The model under review builds one solid part; all positions refer to its coordinate system, in mm. A direction names the side the tool comes from. Coordinates: 2 decimals unless noted, no trailing zeros. Write each loop counter-clockwise with the first axis right and the second up, starting at its lowest first coordinate (ties: lowest second). Pieces come first, ordered by that corner, then holes.
```python
from build123d import *

# Parameters (mm, degrees)
BOSS_EXTRUDE1_DEPTH = 5
CUT_EXTRUDE1_DEPTH  = 3
FILLET2_R           = 1
FILLET3_R           = 1
FILLET4_R           = 3
LPATTERN1_COUNT     = 2
LPATTERN1_PITCH     = 70
BOSS_EXTRUDE2_REACH = 80.869
SKETCH3_W           = 51.273928048
SKETCH3_H           = 5


with BuildPart() as part:
    # Sketch1 → Boss-Extrude1 (new, symmetric)
    with BuildSketch(Plane.XY):
        with BuildLine():
            Line((25.636964024, -25.75), (25.636964024, -2))
            Line((25.636964024, -2), (17.636964024, -2))
            ThreePointArc((17.636964024, -2), (0, -17.75), (-17.636964024, -2))
            Line((-17.636964024, -2), (-25.636964024, -2))
            Line((-25.636964024, -2), (-25.636964024, -25.75))
            Line((-25.636964024, -25.75), (25.636964024, -25.75))
        make_face()
    extrude(amount=BOSS_EXTRUDE1_DEPTH, both=True)

    # Sketch2 → Cut-Extrude1 (cut, symmetric)
    with BuildSketch(Plane.XY):
        Polygon((25.636964024, -2), (21.636964024, -7.712592027), (25.636964024, -18.702501705), align=None)
    cut_extrude1 = extrude(amount=CUT_EXTRUDE1_DEPTH, both=True, mode=Mode.SUBTRACT)

    # Mirror4: Cut-Extrude1 across plane
    add(cut_extrude1.mirror(Plane(origin=(0, 0, 0), x_dir=(0, 0, 1), z_dir=(1, 0, 0))), mode=Mode.SUBTRACT)

    # Fillet2
    fillet2_edges = [part.edges().sort_by_distance(p)[0] for p in [
        (25.636964024, -2, 0),
        (-25.636964024, -2, 0),
    ]]
    fillet(fillet2_edges, radius=FILLET2_R)

    # Fillet3
    fillet3_edges = [part.edges().sort_by_distance(p)[0] for p in [
        (25.636964024, -2, 4),
        (-25.636964024, -2, 4),
        (25.636964024, -2, -4),
        (-25.636964024, -2, -4),
    ]]
    fillet(fillet3_edges, radius=FILLET3_R)

    # Fillet4
    fillet4_edges = [part.edges().sort_by_distance(p)[0] for p in [
        (-17.636964024, -2, 0),
        (17.636964024, -2, 0),
    ]]
    fillet(fillet4_edges, radius=FILLET4_R)


with BuildPart() as lpattern1_1:
    # LPattern1: pattern copy
    add(part.part.moved(Location(Vector(0, 0, 1) * (1 * LPATTERN1_PITCH))))

    # Sketch3 → Boss-Extrude2 (add, up to next)
    with BuildSketch(Plane.XY.offset(5), mode=Mode.PRIVATE) as boss_extrude2_sk1:
        with Locations((0, -23.25)):
            Rectangle(SKETCH3_W, SKETCH3_H)
    boss_extrude2_tool1 = extrude(boss_extrude2_sk1.sketch, amount=BOSS_EXTRUDE2_REACH, mode=Mode.PRIVATE) - lpattern1_1.part

    add(part.part)  # Boss-Extrude2 merges part
    add(boss_extrude2_tool1.solids().sort_by_distance((0, -23.25, 5))[0])


solid = lpattern1_1.part
```
Item 1: Take a section at D-D, the plane x = 9. Write out the cut boundary in (y, z).
Solved:
outline: (-25.75, -5) - (-15.3, -5) - (-15.3, 5) - (-20.75, 5) - (-20.75, 65) - (-15.3, 65) - (-15.3, 75) - (-25.75, 75) - close
Item 2: Take a section at A-A, the plane y = -16.75. Count the separate pieces of the cut face and the enclosed holes in it, plus the area to 3 significant figures.
Solved:
separate pieces: 4
enclosed holes: 0
area: 773 mm2
Item 3: For pin 1 (2 mm diameter, centred on x = -0.5, z = 27, fed in from +Y); pin 2 (1.5 mm diameter, centred on x = 6.5, y = -15.5, fed in from +Z), all flat-tipped, find the tip position at first contact; note any pin that passes through.
Solved:
pin 1: stops at y = -20.75
pin 2: passes through
Item 4: Take a section at B-B, the plane z = 30.5. Write out the cut boundary in (x, y).
Solved:
outline: (-25.64, -25.75) - (25.64, -25.75) - (25.64, -20.75) - (-25.64, -20.75) - close
Item 5: To check wall thickness, follow line 1 along Z through (x, y) = (-21.5, -19.75); line 2 along Z through (x, y) = (-22.5, -8.25); line 3 along Y through (x, z) = (-3.5, 52). State the ranges of each line that lie inside material, in increasing order.
Solved:
line 1: z = -5 to 5, 65 to 75
line 2: z = -5 to -3, 3 to 5, 65 to 67, 73 to 75
line 3: y = -25.75 to -20.75
Item 6: Mouldability with a two-part tool opening along Z and no side actions: class faces 5 (the face through (0, -19, 75)), 6 (the face through (23.11, -5.61, 70.04)), 7 (the face through (-22, -2, 70)) as pulls with the +Z half, pulls with the -Z half, needs draft (parallel to the pull), parting line crosses it, or undercut.
Solved:
face 5: pulls with the +Z half
face 6: undercut
face 7: needs draft
Item 7: Machinability: for faces 1 (the face through (0, -20, 65)), 2 (the face through (18.31, -2.62, 0.07)), 3 (the face through (-24, -10, -3)), 4 (the face through (24.596, -2.525, -0.042)), which of the approach directions +Z, -Z, +X, -X, +Y, -Y give a long, thin tool a straight path to every point of the face, cutting with its end or side? Answer none if there is none.
Solved:
face 1: +X, -X, +Y
face 2: +Z, -Z, +Y
face 3: -X
face 4: +X
